```python
from build123d import *

# Parameters (mm, degrees)
SKETCH2_R           = 37.465
BOSS_EXTRUDE1_DEPTH = 50.8
SKETCH3_R           = 9.525
CUT_REVOLVE1_ANGLE  = 180
SKETCH4_R           = 37.465
SKETCH4_R_2         = 9.525
BOSS_EXTRUDE2_DEPTH = 25.4
SKETCH5_R           = 3.4671
CUT_EXTRUDE1_DEPTH  = 254


with BuildPart() as part:
    # Sketch1 → Revolve1 (revolve)
    with BuildSketch(Plane.XY):
        with BuildLine():
            Line((0, 0), (304.8, 0))
            Line((304.8, 0), (304.8, 39.6748))
            add(Edge.make_bspline(
                [(0, 0), (0.001990016, 0.006380343), (0.00701971, 0.018647451), (0.02144512, 0.041133145), (0.054977521, 0.082482136), (0.104001435, 0.131550788), (0.168386027, 0.187594696), (0.261246618, 0.26037229), (0.388654902, 0.350880875), (0.581878865, 0.475164865), (0.906754263, 0.663154837), (1.458542633, 0.94838722), (2.421507462, 1.387921999), (4.163311697, 2.085133875), (7.330620723, 3.184538925), (12.605144246, 4.765142981), (22.086176793, 7.229960877), (35.434892871, 10.199581229), (51.943243843, 13.427910643), (70.826030727, 16.720256354), (89.756201504, 19.724478891), (108.72270084, 22.489997643), (127.717963157, 25.049113562), (146.737633519, 27.420133683), (165.778389571, 29.614813334), (184.838106864, 31.638406979), (203.915143101, 33.491467662), (223.008423973, 35.16936619), (242.117188184, 36.660980831), (261.241034269, 37.946600905), (277.448292398, 38.829280667), (289.805240869, 39.3397638), (298.30529744, 39.58036416), (302.01635164, 39.649528), (303.872082374, 39.671991977), (304.8, 39.6748)],
                knots=[0, 0, 0, 0, 0, 8.6237e-05, 0.000172473, 0.000344946, 0.000689892, 0.00098475, 0.001279607, 0.001875338, 0.002717212, 0.003964713, 0.006148621, 0.009932249, 0.016447924, 0.028301276, 0.049639613, 0.081363147, 0.143539844, 0.20571656, 0.267893272, 0.330069984, 0.392246696, 0.454423407, 0.516600119, 0.578776833, 0.640953546, 0.703130258, 0.765306971, 0.827483684, 0.889660397, 0.95183711, 0.975918555, 0.987959278, 1, 1, 1, 1, 1], degree=4))
        make_face()
    revolve(axis=Axis((0, 0, 0), (1, 0, 0)))

    # Sketch2 → Boss-Extrude1 (add)
    with BuildSketch(Plane(origin=(304.8, 0, 0), x_dir=(0, 0, -1), z_dir=(1, 0, 0))):
        with Locations(Location((0, 0, 0), (0, 0, 180))):
            Circle(SKETCH2_R)
    extrude(amount=BOSS_EXTRUDE1_DEPTH)

    # Sketch3 → Cut-Revolve1 (revolve, cut)
    with BuildSketch(Plane(origin=(355.6, 0, 0), x_dir=(0, 0, -1), z_dir=(1, 0, 0))):
        with Locations((-19.05, 0)):
            Circle(SKETCH3_R)
    revolve(axis=Axis((355.6, 37.465, 0), (0, -1, 0)), revolution_arc=CUT_REVOLVE1_ANGLE, mode=Mode.SUBTRACT)

    # Sketch4 → Boss-Extrude2 (add)
    with BuildSketch(Plane(origin=(355.6, 0, 0), x_dir=(0, 0, -1), z_dir=(1, 0, 0))):
        with Locations(Location((0, 0, 0), (0, 0, 180))):
            Circle(SKETCH4_R)
        with Locations(Location((-19.05, 0, 0), (0, 0, 180))):
            Circle(SKETCH4_R_2, mode=Mode.SUBTRACT)
        with Locations((19.05, 0)):
            Circle(SKETCH4_R_2, mode=Mode.SUBTRACT)
    extrude(amount=BOSS_EXTRUDE2_DEPTH)

    # Sketch5 → Cut-Extrude1 (cut)
    with BuildSketch(Plane(origin=(381, 0, 0), x_dir=(0, 0, -1), z_dir=(1, 0, 0))):
        with Locations((0, 16.51)):
            Circle(SKETCH5_R)
        with Locations((0, -16.51)):
            Circle(SKETCH5_R)
    extrude(amount=-CUT_EXTRUDE1_DEPTH, mode=Mode.SUBTRACT)


solid = part.part
```
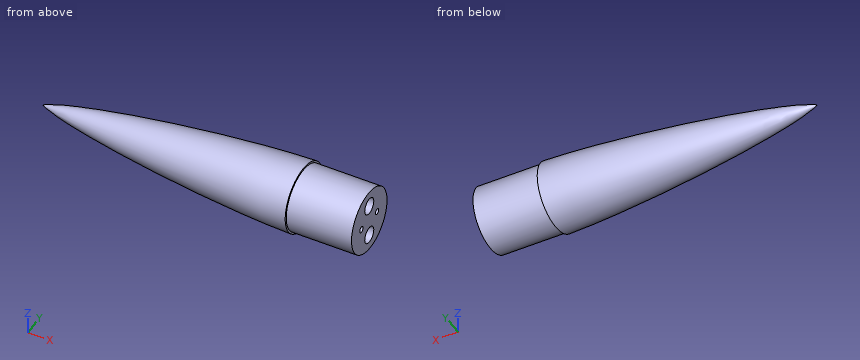
Geometry check sheet. Reference: the model listing, model coordinates, mm. Round coordinates to 2 decimals unless told otherwise and drop trailing zeros. Use a Markdown table: item, result.
(1) Go/stop test with flat-tipped pins: P1, Ø4, axis at y = -16.51, z = 0, coming from the +X side; P2, Ø7.5, axis at y = 16.5, z = 1.5, coming from the +X side; P3, Ø1.5, axis at x = 328.5, y = -15, coming from the -Z side; P4, Ø1.5, axis at x = 298.5, z = -17, coming from the +Y side. Record where each tip stops, or that it passes through.
Calculated:
| item | result |
|---|---|
| P1 | x = 127 |
| P2 | x = 381 |
| P3 | z = -34.65 |
| P4 | y = 36.09 |
(2) Scan lines: probe 1 along Y at (x, z) = (351.5, 26.5); probe 2 along Y at (x, z) = (361.25, 19.05) (3 decimals); probe 3 along Z at (x, y) = (273, 16). Record each from-to range of solid material in increasing order.
Calculated:
| item | result |
|---|---|
| probe 1 | -26.48 to -5.52, 5.52 to 26.48 |
| probe 2 | -32.26 to -9.525, 9.525 to 32.26 |
| probe 3 | -35.08 to -3.43, 3.43 to 35.08 |
(3) Sectioned sample at A-A (x = 335). Give the number of separate pieces and of enclosed holes in the cut face, then the cut area to 3 significant figures.
Calculated:
| item | result |
|---|---|
| separate pieces | 1 |
| enclosed holes | 3 |
| area | 3,710 mm² |
